Geometry check sheet. Reference: the model listing, model coordinates, mm. Face numbers are marked on the shaded views. Give positions to 0.01 mm unless a question says otherwise; leave off trailing zeros. Write each loop counter-clockwise with the first axis right and the second up, starting at its lowest first coordinate (ties: lowest second). Pieces come first, ordered by that corner, then holes. Notation, with made-up numbers: M 83,63 L 97,63 A14 ccw 97,69 Z; hole C 3.5,70.25 d9. An arc over 180 degrees is marked long. One line per item, written item: value. Start each with the question number.
1. Gauge pin test, flat ends, axial feed: pin 1 (2 mm diameter, centred on x = -29, y = 13.5, fed in from -Z); pin 2 (1.5 mm diameter, centred on y = 8.5, z = 2, fed in from +X); pin 3 (2 mm diameter, centred on x = -8, z = -13, fed in from -Y); pin 4 (1.6 mm diameter, centred on y = 14, z = 0, fed in from -X). Record the tip position at first contact, or that the pin passes through.
2. Cross-section at D-D on z = -17. Record the cut outline in (x, y).
3. Cross-section at B-B on y = 7.75. Record the cut outline in (x, z).
4. Cross-section at A-A on z = 0. Record the cut outline in (x, y).
5. Cross-section at C-C on z = 11. Record the cut outline in (x, y).
6. Release check for a two-part mould opening along Z. For the marked faces 1, 2, 3 and 4 record: pulls with the +Z half, pulls with the -Z half, needs draft (parallel to the pull), parting line crosses it, or undercut.
7. Scan lines: line 1 (X direction, y = 1.9, z = 0); line 2 (X direction, y = 11.5, z = 0); line 3 (Z direction, x = -1, y = 10.25). Record each from-to range of solid material in increasing order.
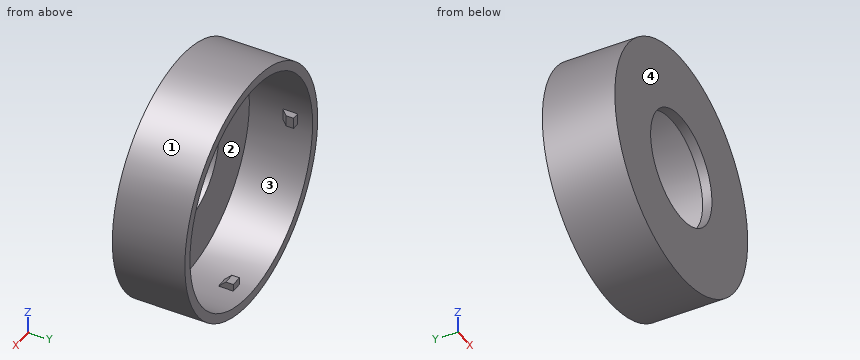
from build123d import *

# Parameters (mm, degrees)
SKETCH1_R           = 32.5
BOSS_EXTRUDE1_DEPTH = 2.5
SKETCH2_R           = 32.5
SKETCH2_R_2         = 30
BOSS_EXTRUDE2_DEPTH = 17
BOSS_EXTRUDE3_START = -2
BOSS_EXTRUDE3_DEPTH = 2
CHAMFER1_SIZE       = 2
SKETCH4_R           = 15
CUT_EXTRUDE1_DEPTH  = 50.005101775


with BuildPart() as part:
    # Sketch1 → Boss-Extrude1 (new body)
    with BuildSketch(Plane(origin=(0, 0, 0), x_dir=(1, 0, 0), z_dir=(0, 1, 0))):
        with Locations(Location((0, 0, 0), (0, 0, 270))):
            Circle(SKETCH1_R)
    extrude(amount=BOSS_EXTRUDE1_DEPTH)

    # Sketch2 → Boss-Extrude2 (add)
    with BuildSketch(Plane(origin=(0, 2.5, 0), x_dir=(1, 0, 0), z_dir=(0, 1, 0))):
        with Locations(Location((0, 0, 0), (0, 0, 270))):
            Circle(SKETCH2_R)
        with Locations(Location((0, 0, 0), (0, 0, 270))):
            Circle(SKETCH2_R_2, mode=Mode.SUBTRACT)
    extrude(amount=BOSS_EXTRUDE2_DEPTH)

    # Sketch3 → Boss-Extrude3 (add)
    with BuildSketch(Plane(origin=(0, 15.5, 0), x_dir=(1, 0, 0), z_dir=(0, 1, 0)).offset(BOSS_EXTRUDE3_START)):
        with BuildLine():
            Line((-1.5, 28), (1.5, 28))
            Line((1.5, 28), (1.5, 29.962476533))
            ThreePointArc((1.5, 29.962476533), (0, 30), (-1.5, 29.962476533))
            Line((-1.5, 29.962476533), (-1.5, 28))
        make_face()
        with BuildLine():
            Line((-28, 1.5), (-29.962476533, 1.5))
            ThreePointArc((-29.962476533, 1.5), (-30, 0), (-29.962476533, -1.5))
            Line((-29.962476533, -1.5), (-28, -1.5))
            Line((-28, -1.5), (-28, 1.5))
        make_face()
        with BuildLine():
            ThreePointArc((30, 0), (29.990617666, 0.750234632), (29.962476533, 1.5))
            Line((29.962476533, 1.5), (28, 1.5))
            Line((28, 1.5), (28, -1.5))
            Line((28, -1.5), (29.962476533, -1.5))
            ThreePointArc((29.962476533, -1.5), (29.990617666, -0.750234632), (30, 0))
        make_face()
        with BuildLine():
            ThreePointArc((-1.5, -29.962476533), (0, -30), (1.5, -29.962476533))
            Line((1.5, -29.962476533), (1.5, -28))
            Line((1.5, -28), (-1.5, -28))
            Line((-1.5, -28), (-1.5, -29.962476533))
        make_face()
    extrude(amount=BOSS_EXTRUDE3_DEPTH)

    # Chamfer1
    # the kernel refuses this chamfer: 2 mm, written as the material it adds along each edge
    with BuildSketch(Plane(origin=(0, 13.5, 0), x_dir=(0, 0, 1), z_dir=(-1, 0, 0))) as chamfer1_piece_1_section:
        Polygon((30, -CHAMFER1_SIZE), (30 - CHAMFER1_SIZE, 0), (30, 0), align=None)
    chamfer1_piece_1 = revolve(axis=Axis((0, 13.5, 0), (0, 1, 0)), revolution_arc=12.689093413, mode=Mode.PRIVATE)
    chamfer1_piece_1 = split(chamfer1_piece_1, bisect_by=Plane(origin=(1.5, 12.838755732, 29.330774017), z_dir=(-1, 0, 0)), keep=Keep.TOP, mode=Mode.PRIVATE)
    chamfer1_piece_1 = split(chamfer1_piece_1, bisect_by=Plane(origin=(0.749919513, 12.838755732, 28), z_dir=(0, 0, 1)), keep=Keep.TOP, mode=Mode.PRIVATE)
    add(chamfer1_piece_1)
    with BuildSketch(Plane(origin=(0, 13.5, 0), x_dir=(0.9755763292717098, 0, 0.21966070600982865), z_dir=(-0.21966070600982865, 0, 0.9755763292717098))) as chamfer1_piece_2_section:
        Polygon((30, -CHAMFER1_SIZE), (30 - CHAMFER1_SIZE, 0), (30, 0), align=None)
    chamfer1_piece_2 = revolve(axis=Axis((0, 13.5, 0), (0, 1, 0)), revolution_arc=25.378210829, mode=Mode.PRIVATE)
    chamfer1_piece_2 = split(chamfer1_piece_2, bisect_by=Plane(origin=(29.330774007, 12.838755737, 1.5), z_dir=(0, 0, -1)), keep=Keep.TOP, mode=Mode.PRIVATE)
    chamfer1_piece_2 = split(chamfer1_piece_2, bisect_by=Plane(origin=(29.330774007, 12.838755737, -1.5), z_dir=(0, 0, 1)), keep=Keep.TOP, mode=Mode.PRIVATE)
    chamfer1_piece_2 = split(chamfer1_piece_2, bisect_by=Plane(origin=(28, 12.838755737, 0), z_dir=(1, 0, 0)), keep=Keep.TOP, mode=Mode.PRIVATE)
    add(chamfer1_piece_2)
    with BuildSketch(Plane(origin=(0, 13.5, 0), x_dir=(0.21966070600991422, 0, -0.9755763292716906), z_dir=(0.9755763292716906, 0, 0.21966070600991422))) as chamfer1_piece_3_section:
        Polygon((30, -CHAMFER1_SIZE), (30 - CHAMFER1_SIZE, 0), (30, 0), align=None)
    chamfer1_piece_3 = revolve(axis=Axis((0, 13.5, 0), (0, 1, 0)), revolution_arc=25.378210829, mode=Mode.PRIVATE)
    chamfer1_piece_3 = split(chamfer1_piece_3, bisect_by=Plane(origin=(1.5, 12.838755737, -29.330774007), z_dir=(-1, 0, 0)), keep=Keep.TOP, mode=Mode.PRIVATE)
    chamfer1_piece_3 = split(chamfer1_piece_3, bisect_by=Plane(origin=(-1.5, 12.838755737, -29.330774007), z_dir=(1, 0, 0)), keep=Keep.TOP, mode=Mode.PRIVATE)
    chamfer1_piece_3 = split(chamfer1_piece_3, bisect_by=Plane(origin=(0, 12.838755737, -28), z_dir=(0, 0, -1)), keep=Keep.TOP, mode=Mode.PRIVATE)
    add(chamfer1_piece_3)
    with BuildSketch(Plane(origin=(0, 13.5, 0), x_dir=(-0.9755763292716926, 0, -0.21966070600990492), z_dir=(0.21966070600990492, 0, -0.9755763292716926))) as chamfer1_piece_4_section:
        Polygon((30, -CHAMFER1_SIZE), (30 - CHAMFER1_SIZE, 0), (30, 0), align=None)
    chamfer1_piece_4 = revolve(axis=Axis((0, 13.5, 0), (0, 1, 0)), revolution_arc=25.378210829, mode=Mode.PRIVATE)
    chamfer1_piece_4 = split(chamfer1_piece_4, bisect_by=Plane(origin=(-29.330774007, 12.838755737, -1.5), z_dir=(0, 0, 1)), keep=Keep.TOP, mode=Mode.PRIVATE)
    chamfer1_piece_4 = split(chamfer1_piece_4, bisect_by=Plane(origin=(-29.330774007, 12.838755737, 1.5), z_dir=(0, 0, -1)), keep=Keep.TOP, mode=Mode.PRIVATE)
    chamfer1_piece_4 = split(chamfer1_piece_4, bisect_by=Plane(origin=(-28, 12.838755737, 0), z_dir=(-1, 0, 0)), keep=Keep.TOP, mode=Mode.PRIVATE)
    add(chamfer1_piece_4)
    with BuildSketch(Plane(origin=(0, 13.5, 0), x_dir=(-0.2196605016666056, 0, 0.9755763752815949), z_dir=(-0.9755763752815949, 0, -0.2196605016666056))) as chamfer1_piece_5_section:
        Polygon((30, -CHAMFER1_SIZE), (30 - CHAMFER1_SIZE, 0), (30, 0), align=None)
    chamfer1_piece_5 = revolve(axis=Axis((0, 13.5, 0), (0, 1, 0)), revolution_arc=12.689093413, mode=Mode.PRIVATE)
    chamfer1_piece_5 = split(chamfer1_piece_5, bisect_by=Plane(origin=(-1.5, 12.838755737, 29.330774007), z_dir=(1, 0, 0)), keep=Keep.TOP, mode=Mode.PRIVATE)
    chamfer1_piece_5 = split(chamfer1_piece_5, bisect_by=Plane(origin=(-0.749919511, 12.838755737, 28), z_dir=(0, 0, 1)), keep=Keep.TOP, mode=Mode.PRIVATE)
    add(chamfer1_piece_5)

    # Sketch4 → Cut-Extrude1 (cut, through all)
    with BuildSketch(Plane(origin=(0, 2.5, 0), x_dir=(1, 0, 0), z_dir=(0, 1, 0))):
        with Locations(Location((0, 0, 0), (0, 0, 270))):
            Circle(SKETCH4_R)
    extrude(amount=-CUT_EXTRUDE1_DEPTH, mode=Mode.SUBTRACT)


solid = part.part
Report:
1. pin 1: stops at z = -16.5
1. pin 2: stops at x = 32.48
1. pin 3: stops at y = 0
1. pin 4: stops at x = -32.5
2. outline: M -27.7,0 L 27.7,0 L 27.7,19.5 L 24.72,19.5 L 24.72,2.5 L -24.72,2.5 L -24.72,19.5 L -27.7,19.5 Z
3. outline: C 0,0 d65; hole C 0,0 d60
4. outline: M -32.5,0 L -15,0 L -15,2.5 L -30,2.5 L -30,11.5 L -28,13.5 L -28,15.5 L -30,15.5 L -30,19.5 L -32.5,19.5 Z; M 15,0 L 32.5,0 L 32.5,19.5 L 30,19.5 L 30,15.5 L 28,15.5 L 28,13.5 L 30,11.5 L 30,2.5 L 15,2.5 Z
5. outline: M -30.58,0 L -10.2,0 L -10.2,2.5 L -27.91,2.5 L -27.91,19.5 L -30.58,19.5 Z; M 10.2,0 L 30.58,0 L 30.58,19.5 L 27.91,19.5 L 27.91,2.5 L 10.2,2.5 Z
6. face 1: parting line crosses it
6. face 2: undercut
6. face 3: undercut
6. face 4: needs draft
7. line 1: x = -32.5 to -15, 15 to 32.5
7. line 2: x = -32.5 to -30, 30 to 32.5
7. line 3: z = -32.48 to -29.98, 29.98 to 32.48
